Here's the drawing with two shaded views (mm, measured from the low corner). I have some questions. A direction names the side the tool comes from. Give positions to 0.01 mm unless a question says otherwise; leave off trailing zeros. Order: outer loops, then holes, each group sorted by start corner. A loop starts at its lowest first (then second) coordinate and runs counter-clockwise, first axis right, second up. Notation, with made-up numbers: M 23,18.25 L 80,18.25 A18 ccw 80,43.25 Z; hole C 73,-35.5 d3. An arc over 180 degrees is marked long. Use a Markdown table: item, result. Add a question column.
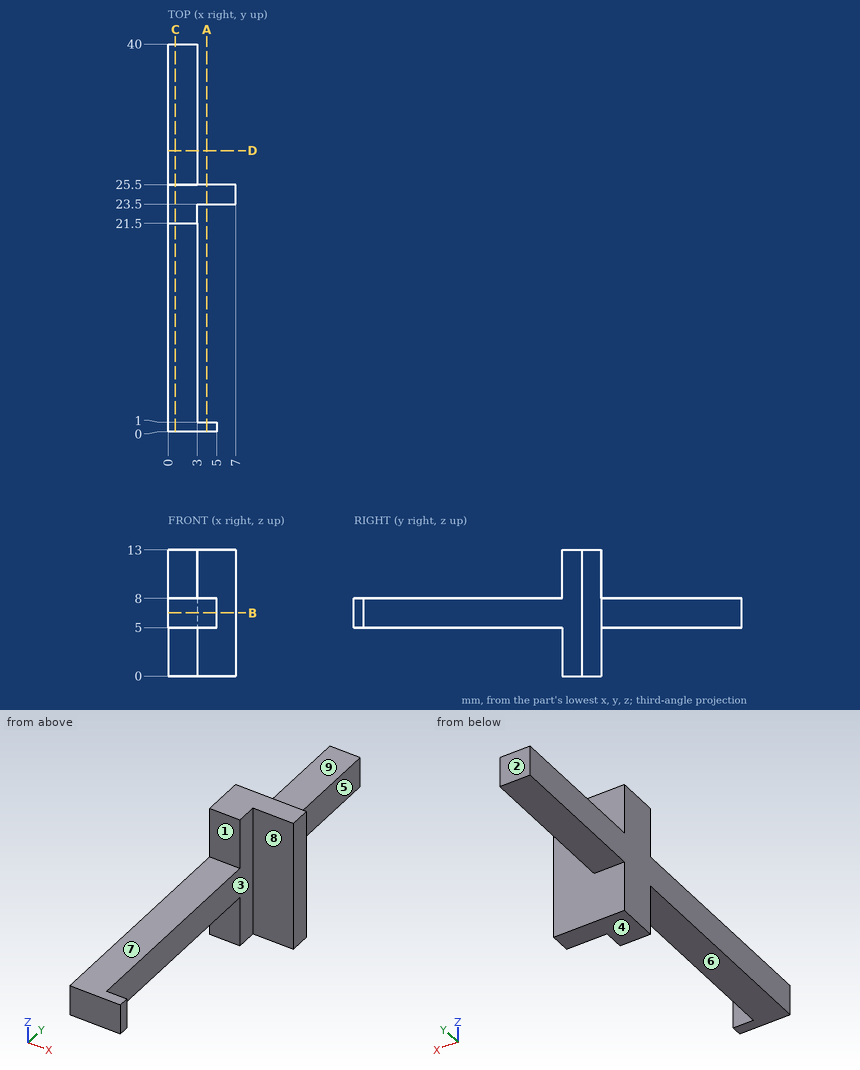
1) Suppose I cut it at A-A on x = 4. Please give me the cut outline in (y, z), and give its area (3 significant figures).
2) We'd pull the mould along Y, two halves only. Please class the marked faces 1, 2, 3 and 4: pulls with the +Y half, pulls with the -Y half, needs draft (parallel to the pull), parting line crosses it, or undercut.
3) For the marked faces 5, 6, 7, 8 and 9, which set-ups out of +Z, -Z, +X, -X, +Y, -Y let a thin tool reach every point of the face, with its end or its side?
4) Suppose I cut it at C-C on x = 0.75. Please give me the cut outline in (y, z).
5) For pin 1 (1.5 mm diameter, centred on x = 2, z = 11.5, fed in from -Y); pin 2 (5 mm diameter, centred on y = 29, z = 10, fed in from +X); pin 3 (1.5 mm diameter, centred on x = 1.5, y = 10, fed in from -Z), each with a flat end and sliding along its axis, tell me the tip position at first contact or that it passes through.
6) Suppose I cut it at B-B on z = 6.5. Please give me the cut outline in (x, y), and give its area (3 significant figures).
7) Suppose I cut it at D-D on y = 29. Please give me the cut outline in (x, z), and give its area (3 significant figures).
8) Please list where these lines run through material, in increasing order: line 1 (X direction, y = 38, z = 6.5); line 2 (Z direction, x = 2.25, y = 7); line 3 (Y direction, x = 4.25, z = 2.25). Write a range as from..to.
Values found:
| question | item | result |
|---|---|---|
| 1 | outline | M 0,5 L 1,5 L 1,8 L 0,8 Z; M 23.5,0 L 25.5,0 L 25.5,13 L 23.5,13 Z |
| 1 | area | 29.0 mm^2 |
| 2 | face 1 | pulls with the -Y half |
| 2 | face 2 | pulls with the +Y half |
| 2 | face 3 | undercut |
| 2 | face 4 | needs draft |
| 3 | face 5 | +Z, -Z, +X, +Y |
| 3 | face 6 | -Z, +X, -X, -Y |
| 3 | face 7 | +Z, +X, -X, -Y |
| 3 | face 8 | +Z, -Z, +X |
| 3 | face 9 | +Z, +X, -X, +Y |
| 4 | outline | M 0,5 L 21.5,5 L 21.5,0 L 25.5,0 L 25.5,5 L 40,5 L 40,8 L 25.5,8 L 25.5,13 L 21.5,13 L 21.5,8 L 0,8 Z |
| 5 | pin 1 | stops at y = 21.5 |
| 5 | pin 2 | stops at x = 3 |
| 5 | pin 3 | stops at z = 5 |
| 6 | outline | M 0,0 L 5,0 L 5,1 L 3,1 L 3,23.5 L 7,23.5 L 7,25.5 L 3,25.5 L 3,40 L 0,40 Z |
| 6 | area | 130 mm^2 |
| 7 | outline | M 0,5 L 3,5 L 3,8 L 0,8 Z |
| 7 | area | 9.00 mm^2 |
| 8 | line 1 | x = 0..3 |
| 8 | line 2 | z = 5..8 |
| 8 | line 3 | y = 23.5..25.5 |
